Verification items for the finished model (mm, model axes). A direction names the side the tool comes from. Give positions to 0.01 mm unless a question says otherwise; leave off trailing zeros. Write each loop counter-clockwise with the first axis right and the second up, starting at its lowest first coordinate (ties: lowest second). Pieces come first, ordered by that corner, then holes. Notation, with made-up numbers: (47, 9.5) -> (97, 9.5) arc R36 cw to (97, 48.5) -> close; hole circle Ø11 at (3.25, 12). An arc over 180 degrees is marked (long way). Write item = value, one per line.
from build123d import *

# Parameters (mm, degrees)
F0_W     = 100.4092097282
F0_H     = 89.206546545
F1_DEPTH = 97.7773964405
F2_R     = 22.0167060196
F2_R_2   = 21.115809679
F3_DEPTH = 114.1652464867
F4_R     = 5.08
F5_R     = 33.8357748328
F6_DEPTH = 98.3386710286
F7_R     = 5


# Not quite as in the source:
# - a fillet or chamfer that OpenCascade refuses, or shapes differently, is made with other operations: its cross-section is extruded or revolved along the edge and cut away or added
# - the program builds the solid bodies; features that only make, move or delete a surface that nothing else refers to are left out


with BuildPart() as f1:
    # F0 (on Front) → F1 (new body)
    with BuildSketch(Plane.XZ):
        Rectangle(F0_W, F0_H)
    extrude(amount=F1_DEPTH)

    # F2 (on Top) → F3 (join)
    with BuildSketch(Plane.XY):
        with Locations((0, -40.3943955898)):
            Circle(F2_R)
        with Locations((0, -40.3943955898)):
            Circle(F2_R_2, mode=Mode.SUBTRACT)
    extrude(amount=F3_DEPTH)

    # F4
    f4_edges = [f1.edges().sort_by_distance(p)[0] for p in [
        (50.204605, -48.888698, 44.603273),
        (0, 0, 44.603273),
        (0, -97.777396, 44.603273),
        (-50.204605, -48.888698, 44.603273),
        (-22.016706, -40.394396, 44.603273),
        (0, -97.777396, -44.603273),
        (50.204605, -97.777396, 0),
        (-50.204605, -97.777396, 0),
        (-50.204605, -48.888698, -44.603273),
        (-50.204605, 0, 0),
        (50.204605, -48.888698, -44.603273),
        (50.204605, 0, 0),
    ]]
    fillet(f4_edges, radius=F4_R)

    # F5 (on Front) → F6 (cut)
    with BuildSketch(Plane.XZ):
        Circle(F5_R)
    extrude(amount=F6_DEPTH, mode=Mode.SUBTRACT)

    # F7
    f7_edges = [f1.edges().sort_by_distance(p)[0] for p in [
        (50.204605, -48.888698, 39.523273),
        (50.204605, -5.08, 0),
        (50.204605, -92.697396, 0),
        (50.204605, -48.888698, -39.523273),
        (-33.835775, -97.777396, 0),
    ]]
    fillet(f7_edges, radius=F7_R)

    # F10: fillet of radius 10 on 1 edges, made by hand

    # F10_s1 → F10_t2 (revolve, cut)
    with BuildSketch(Plane.XZ.offset(40.3943955898)):
        with BuildLine():
            ThreePointArc((22.0167060196, 110.017197235), (21.7888868559, 112.1395736631), (21.115809679, 114.1652464867))
            Line((21.115809679, 114.1652464867), (22.0167060196, 114.1652464867))
            Line((22.0167060196, 114.1652464867), (22.0167060196, 110.017197235))
        make_face()
    revolve(axis=Axis((0, -40.3943955898, 114.1652464867), (0, 0, 1)), mode=Mode.SUBTRACT)


solid = f1.part
Item 1: Set-up check for faces 1 (the cylindrical face through (48.756, -46.998, -43.076)), 2 (the cylindrical face through (21, -33.78, 79.43)): record each of +Z, -Z, +X, -X, +Y, -Y from which the full face is reachable in a straight line by a thin tool's end or side.
Response values:
face_1 = -Z, +X, +Y, -Y
face_2 = +Z
Item 2: Sectioned sample at B-B on z = 0. Record the cut outline in (x, y).
Response values:
outline = (-50.2, -92.7) arc R5.08 ccw to (-45.12, -97.78) -> (-38.84, -97.78) arc R5 ccw to (-33.84, -92.78) -> (-33.84, 0) -> (-45.12, 0) arc R5.08 ccw to (-50.2, -5.08) -> close; (33.84, -92.78) arc R5 ccw to (38.84, -97.78) -> (45.12, -97.78) arc R5.08 ccw to (50.2, -92.7) -> (50.2, -5.08) arc R5.08 ccw to (45.12, 0) -> (33.84, 0) -> close
Item 3: Sectioned sample at A-A on x = 0. Record the cut outline in (y, z), then the cut area to 3 significant figures.
Response values:
outline = (-97.78, -39.52) arc R5.08 ccw to (-92.7, -44.6) -> (0, -44.6) -> (0, -33.84) -> (-92.78, -33.84) arc R5 ccw to (-97.78, -38.84) -> close; (-97.78, 38.84) arc R5 ccw to (-92.78, 33.84) -> (0, 33.84) -> (0, 39.52) arc R5.08 ccw to (-5.08, 44.6) -> (-13.3, 44.6) arc R5.08 cw to (-18.38, 49.68) -> (-18.38, 110.02) arc R10 ccw to (-19.28, 114.17) -> (-19.28, 44.6) -> (-61.51, 44.6) -> (-61.51, 114.17) arc R10 ccw to (-62.41, 110.02) -> (-62.41, 49.68) arc R5.08 cw to (-67.49, 44.6) -> (-92.7, 44.6) arc R5.08 ccw to (-97.78, 39.52) -> close
area = 2,210 mm^2
Item 4: Sectioned sample at C-C on y = -75.5. Record the cut outline in (x, z), then the cut area to 3 significant figures.
Response values:
outline = (-50.2, -39.52) arc R5.08 ccw to (-45.12, -44.6) -> (45.12, -44.6) arc R5.08 ccw to (50.2, -39.52) -> (50.2, 39.52) arc R5.08 ccw to (45.12, 44.6) -> (-45.12, 44.6) arc R5.08 ccw to (-50.2, 39.52) -> close; hole circle Ø67.67 at (0, 0)
area = 5,340 mm^2
Item 5: Sectioned sample at D-D on x = -41. Record the cut outline in (y, z).
Response values:
outline = (-97.78, -39.52) arc R5.08 ccw to (-92.7, -44.6) -> (0, -44.6) -> (0, 39.52) arc R5.08 ccw to (-5.08, 44.6) -> (-92.7, 44.6) arc R5.08 ccw to (-97.78, 39.52) -> close
Item 6: Mould release check, pull along X, two halves, no side actions. Record for faces 3 (the cylindrical face through (20.14, -34.05, 78.9)), 4 (the cylindrical face through (-48.756, -46.998, -43.076)), 5 (the flat face through (19, 0, -30)): +X half, -X half, draft (parallel to the pull), parting line (faces both ways), or undercut.
Response values:
face_3 = undercut
face_4 = -X half
face_5 = draft
Item 7: Material ranges on line 1 (Z direction, x = 0, y = -50.5); line 2 (Y direction, x = 0, z = 96); line 3 (Z direction, x = 39.5, y = -28.5), recorded low to high.
Response values:
line_1 = -44.6 to -33.84, 33.84 to 44.6
line_2 = -62.41 to -61.51, -19.28 to -18.38
line_3 = -44.6 to 44.6
Item 8: Go/stop test with flat-tipped pins: P1, Ø8, axis at y = -46, z = 58.5, coming from the -X side; P2, Ø4, axis at x = -20, y = -16, coming from the +Z side; P3, Ø8, axis at x = -14.5, z = 76, coming from the +Y side. Record where each tip stops, or that it passes through.
Response values:
P1 = -21.96
P2 = 44.6
P3 = -21.04
